Can you work these out from the model? Positions are in its coordinate system, mm. A direction names the side the tool comes from. Coordinates: 2 decimals unless noted, no trailing zeros. Write each loop counter-clockwise with the first axis right and the second up, starting at its lowest first coordinate (ties: lowest second). Pieces come first, ordered by that corner, then holes.
```python
from build123d import *

# Parameters (mm, degrees)
F1_DEPTH = 10
F2_R     = 5
F3_R     = 0.49999


# Not quite as in the source:
# - a fillet or chamfer is up to 0.001 mm smaller than in the source, because OpenCascade refuses the exact size


with BuildPart() as f1:
    # F0 (on Top) → F1 (new body)
    with BuildSketch(Plane.XY):
        with BuildLine():
            ThreePointArc((-1.1283685941, -2.7256713514), (-1.6391785515, 2.4526707232), (2.95, 0))
            ThreePointArc((2.95, 0), (3.035057777, 1.107295327), (3.2882352941, 2.1886088391))
            ThreePointArc((3.2882352941, 2.1886088391), (-2.5695330315, 3), (-2.6678904245, -2.9128784188))
            Line((-2.6678904245, -2.9128784188), (-1.1283685941, -2.7256713514))
        make_face()
        with BuildLine():
            ThreePointArc((3.2882352941, 2.1886088391), (3.035057777, 1.107295327), (2.95, 0))
            ThreePointArc((2.95, 0), (3.035057777, -1.107295327), (3.2882352941, -2.1886088391))
            ThreePointArc((3.2882352941, -2.1886088391), (3.7809409815, -1.1432345753), (3.95, 0))
            ThreePointArc((3.95, 0), (3.7809409815, 1.1432345753), (3.2882352941, 2.1886088391))
        make_face()
        with BuildLine():
            ThreePointArc((3.2882352941, -2.1886088391), (3.035057777, -1.107295327), (2.95, 0))
            ThreePointArc((2.95, 0), (2.6326037224, -1.3311264557), (1.7487134637, -2.3758159065))
            Line((1.7487134637, -2.3758159065), (3.2882352941, -2.1886088391))
        make_face()
        with BuildLine():
            ThreePointArc((3.95, 0), (3.7809409815, -1.1432345753), (3.2882352941, -2.1886088391))
            Line((3.2882352941, -2.1886088391), (4.4925851142, -2.5471386536))
            ThreePointArc((4.4925851142, -2.5471386536), (4.0871511128, -1.3021438023), (3.95, 0))
        make_face()
        with BuildLine():
            ThreePointArc((17.45, 0), (11.307295327, 7.164942223), (3.2882352941, 2.1886088391))
            ThreePointArc((3.2882352941, 2.1886088391), (3.7809409815, 1.1432345753), (3.95, 0))
            ThreePointArc((3.95, 0), (10.2, 6.25), (16.45, 0))
            ThreePointArc((16.45, 0), (15.6872207282, -2.9921411532), (13.5850692222, -5.2539324663))
            Line((13.5850692222, -5.2539324663), (14.7894190423, -5.6124622809))
            ThreePointArc((14.7894190423, -5.6124622809), (16.7511750113, -3.1055765925), (17.45, 0))
        make_face()
    extrude(amount=F1_DEPTH)

    # F2
    f2_edges = [f1.edges().sort_by_distance(p)[0] for p in [
        (3.288235, 2.188609, 5),
    ]]
    fillet(f2_edges, radius=F2_R)

    # F3 (radius 0.5 in the source; OpenCascade refuses exactly that, so slightly less here)
    f3_edges = [f1.edges().sort_by_distance(p)[0] for p in [
        (-1.128369, -2.725671, 5),
        (1.748713, -2.375816, 5),
        (4.492585, -2.547139, 5),
        (13.585069, -5.253932, 5),
        (-2.66789, -2.912878, 5),
    ]]
    fillet(f3_edges, radius=F3_R)


solid = f1.part
```
1. If I drill on L1, parallel to X at y = 1, z = 0.5; L2, parallel to X at y = 0.5, z = 8; L3, parallel to Y at x = 0, z = 7.25, over which ranges is the centre line in solid material (lowest first)?
2. If we section it at C-C, the plane y = -3.5: List the corners of the cut face in (x, z) for me, plus the area to 3 significant figures.
3. I'm going to push flat-ended pins straight in: P1, Ø1.5, axis at x = 1.5, z = 7, coming from the -Y side; P2, Ø5, axis at x = 11.5, z = 6, coming from the -Y side; P3, Ø2, axis at x = 1, z = 7.5, coming from the +Y side. Where does each tip first touch, or does it pass through?
4. If we section it at A-A, the plane y = 5.5: List the corners of the cut face in (x, z) for me.
5. If we section it at B-B, the plane x = -0.25: List the corners of the cut face in (y, z) for me.
6. Which directions (+Z, -Z, +X, -X, +Y, -Y) give clear straight access to the entire face, cutting with the end or side of a thin tool? Please do faces 1 (the face through (4, 2, 0)), 2 (the face through (-2.02, -2.56, 5.07)).
Answers:
1. L1: x = -3.82 to -2.78, 2.78 to 4.03, 16.37 to 17.38
1. L2: x = -3.92 to -2.91, 2.91 to 3.97, 16.43 to 17.43
1. L3: y = 2.95 to 3.95
2. outline: (15.38, 0) - (16.55, 0) - (16.55, 10) - (15.38, 10) - close
2. area: 11.7 mm2
3. P1: stops at y = 1.91
3. P2: stops at y = 4.96
3. P3: stops at y = 3.95
4. outline: (5.48, 0) - (7.23, 0) - (7.23, 10) - (5.48, 10) - close; (13.17, 0) - (14.92, 0) - (14.92, 10) - (13.17, 10) - close
5. outline: (2.94, 0) - (3.94, 0) - (3.94, 10) - (2.94, 10) - close
6. face 1: -Z, +X, -X, +Y, -Y
6. face 2: +Z, -Z
